from build123d import *

# Parameters (mm, degrees)
SKETCH1_W           = 110
SKETCH1_H           = 70
BOSS_EXTRUDE1_DEPTH = 5
BOSS_EXTRUDE2_DEPTH = 5
BOSS_EXTRUDE3_DEPTH = 5
BOSS_EXTRUDE4_START = -70
SKETCH4_R           = 2
BOSS_EXTRUDE4_DEPTH = 70


with BuildPart() as part:
    # Sketch1 → Boss-Extrude1 (new body)
    with BuildSketch(Plane(origin=(0, 0, 0), x_dir=(1, 0, 0), z_dir=(0, 1, 0))):
        Rectangle(SKETCH1_W, SKETCH1_H)
    extrude(amount=BOSS_EXTRUDE1_DEPTH)

    # Sketch2 → Boss-Extrude2 (add)
    with BuildSketch(Plane.XY.offset(35)):
        Polygon((69.722431864, 32), (73.186533479, 30), (55.866025404, 0), (55, 0), (55, 5), (54.133974596, 5), align=None)
    extrude(amount=-BOSS_EXTRUDE2_DEPTH)

    # Sketch3 → Boss-Extrude3 (add)
    with BuildSketch(Plane(origin=(0, 0, -35), x_dir=(-1, 0, 0), z_dir=(0, 0, -1))):
        Polygon((-54.133974596, 5), (-69.722431864, 32), (-73.186533479, 30), (-55.866025404, 0), (-55, 0), (-55, 5), align=None)
    extrude(amount=-BOSS_EXTRUDE3_DEPTH)

    # Sketch4 → Boss-Extrude4 (add)
    with BuildSketch(Plane.XY.offset(35).offset(BOSS_EXTRUDE4_START)):
        with Locations(Location((71.454482672, 31, 0), (0, 0, 330))):
            Circle(SKETCH4_R)
    extrude(amount=BOSS_EXTRUDE4_DEPTH)


solid = part.part
Verification items for the finished model (mm, model axes). A direction names the side the tool comes from. Give positions to 0.01 mm unless a question says otherwise; leave off trailing zeros. Write each loop counter-clockwise with the first axis right and the second up, starting at its lowest first coordinate (ties: lowest second). Pieces come first, ordered by that corner, then holes. Notation, with made-up numbers: M 89.5,68.25 L 99.5,68.25 A15 cw 99.5,92.25 Z; hole C 34.25,62.25 d2. An arc over 180 degrees is marked long. Put each result on its own line as item: value. Start each with the question number.
1. Section check C-C (x = 52). Record the cut outline in (y, z).
2. Section check B-B (y = 21). Record the cut outline in (x, z).
3. Scan lines: line 1 along X through (y, z) = (4, -2); line 2 along Y through (x, z) = (-13, 32.5); line 3 along Y through (x, z) = (66, -32). Record each from-to range of solid material in increasing order. Write a range as [from, to].
4. Set-up check for faces 1 (the face through (10, 4, 35)), 2 (the face through (55, 2, 0)): record each of +Z, -Z, +X, -X, +Y, -Y from which the full face is reachable in a straight line by a thin tool's end or side.
5. Draft check along Z on faces 3 (the face through (72.22, 32.847, -0.49)), 4 (the face through (64.648, 15.21, -32.535)), 5 (the face through (10, 4, -35)). Enter one of: +Z half, -Z half, draft (parallel to the pull), parting line (faces both ways), or undercut.
6. Go/stop test with flat-tipped pins: pin 1 Ø8 at (x, z) = (-26, -11) entering from +Y; pin 2 Ø2.5 at (y, z) = (3, 12) entering from +X. Record where each tip stops, or that it passes through.
7. Section check A-A (z = 28). Record the cut outline in (x, y).
Answer list:
1. outline: M 0,-35 L 5,-35 L 5,35 L 0,35 Z
2. outline: M 63.37,-35 L 67.99,-35 L 67.99,-30 L 63.37,-30 Z; M 63.37,30 L 67.99,30 L 67.99,35 L 63.37,35 Z
3. line 1: [-55, 55]
3. line 2: [0, 5]
3. line 3: [17.55, 25.55]
4. face 1: +Z, +X, -X, +Y, -Y
4. face 2: +X, +Y, -Y
5. face 3: undercut
5. face 4: draft
5. face 5: -Z half
6. pin 1: y = 5
6. pin 2: x = 55
7. outline: M -55,0 L 55,0 L 55,5 L -55,5 Z; C 71.45,31 d4
